Autodesk Inventor part; units mm, degrees
ref_plane "YZ Plane" through (0, 0, 0) normal (1, 0, 0) x (0, 1, 0)
ref_plane "XZ Plane" through (0, 0, 0) normal (0, 1, 0) x (-1, 0, 0)
ref_plane "XY Plane" through (0, 0, 0) normal (0, 0, 1) x (1, 0, 0)
sketch "Sketch1" plane through (0, 0, 0) normal (0, 0, 1) x (1, 0, 0)
  line L0 (0, 0) -> (0, 8)
  line L1 (9, 0) -> (9, 2.5)
  line L2 (9, 2.5) -> (10, 2.5)
  line L3 (10, 2.5) -> (10, 8)
  line L4 (10, 8) -> (12, 8)
  line L5 (12, 8) -> (12, 4.5)
  line L6 (12, 4.5) -> (14, 4.5)
  line L7 (14, 4.5) -> (14, 0)
  line L8 (14, 0) -> (9, 0)
  line L9 (12, 8) -> (15.75, 8)
  line L10 (15.75, 8) -> (15.75, 6.5)
  line L11 (15.75, 6.5) -> (12, 6.5)
  dimension "d0" = 18
  dimension "d2" = 2
  dimension "d3" = 2
  dimension "d4" = 4.5
  dimension "d5" = 20
  dimension "d13" = 28
  dimension "d14" = 1.5
  dimension "d15" = 31.5
  dimension "d28" = 2
revolve "Revolution1" add sketch "Sketch1" angle 360 about axis through (0, 0, 0) along (0, 1, 0)
chamfer "Chamfer1" distance 0.5 angle 45 2 edges at (-14, 4.5, 0) (-14, 0, 0)
thread "Thread1"
sketch "Sketch3" plane through (0, 8, 0) normal (0, 1, 0) x (1, 0, 0)
  circle A0 centre (0, 0) radius 15.75
  circle A1 centre (0, 0) radius 12
  line L0 (12, 0) -> (15.75, 0)
  point P0 (13.875, 0)
hole "Hole2" at (13.875, 8, 0) direction (0, -1, 0) diameter 2.459 depth 1.5
pattern_circular "Circular Pattern2" count 4 over 360 about axis through (0, 5.25, 0) along (0, -1, 0) of "Hole2"
equation "\"d3\" = d2"
properties part number "018"
Could you check a few things on this model? Use its own coordinates, in mm. A direction names the side the tool comes from. Give positions to 0.01 mm unless a question says otherwise; leave off trailing zeros. Order: outer loops, then holes, each group sorted by start corner. A loop starts at its lowest first (then second) coordinate and runs counter-clockwise, first axis right, second up.
1. Will these pins go through, and if not, where does the flat tip stop? P1, Ø4, axis at x = -1.5, z = 7, coming from the +Y side; P2, Ø2, axis at y = 4, z = -9.5, coming from the -X side; P3, Ø1, axis at y = 3, z = -3, coming from the -X side (3 decimals).
2. We'd pull the mould along Z, two halves only. Please class faces 1 (the cylindrical face through (-2.17, 5.29, 9.76)), 2 (the cylindrical face through (-11.99, 5.49, 0.53)), 3 (the flat face through (9, 0, 3)): pulls with the +Z half, pulls with the -Z half, needs draft (parallel to the pull), parting line crosses it, or undercut.
3. Suppose I cut it at A-A (x = 0). Give the number of separate pieces and of enclosed holes in the cut face, plus the area to 3 significant figures.
4. For faces 4 (the cylindrical face through (-1.172, 1.268, -8.923)), 5 (the cylindrical face through (12.932, 2.226, -5.362)), 6 (the cylindrical face through (-0.16, 7.24, -12.656)), 7 (the flat face through (-6, 6.5, -11)), which set-ups out of +Z, -Z, +X, -X, +Y, -Y let a thin tool reach every point of the face, with its end or its side?
5. I need wall thicknesses on L1, parallel to Z at x = 0, y = 6.75; L2, parallel to Z at x = 0, y = 3.65; L3, parallel to Y at x = 9.5, z = -8.5. Which ranges of each line are inside material? Lowest first, please.
6. Suppose I cut it at C-C (y = 6). List the corners of the cut face in (x, z) for me.
Solved:
1. P1: stops at y = 2.5
1. P2: stops at x = -11.12
1. P3: stops at x = -13.775
2. face 1: undercut
2. face 2: parting line crosses it
2. face 3: needs draft
3. separate pieces: 4
3. enclosed holes: 0
3. area: 58.4 mm2
4. face 4: +Y, -Y
4. face 5: -Y
4. face 6: +Y
4. face 7: none
5. L1: z = -15.75 to -15.1, -12.65 to -10, 10 to 12.65, 15.1 to 15.75
5. L2: z = -14 to -10, 10 to 14
5. L3: y = 0 to 4.5, 6.5 to 8
6. outline: circle Ø24 at (0, 0); hole circle Ø20 at (0, 0)
